```python
from build123d import *

# Parameters (mm, degrees)
SKETCH1_R           = 7.5
SKETCH1_R_2         = 4.1
BOSS_EXTRUDE1_DEPTH = 45
SKETCH2_R           = 6.75
SKETCH2_R_2         = 4.5
CUT_EXTRUDE2_DEPTH  = 0.75
CUT_EXTRUDE3_START  = -0.75
SKETCH3_R           = 7
SKETCH3_R_2         = 4.5
CUT_EXTRUDE3_DEPTH  = 0.75
SKETCH4_W           = 0.25
SKETCH4_H           = 1
SKETCH5_W           = 0.25
SKETCH5_H           = 1


with BuildPart() as part:
    # Sketch1 → Boss-Extrude1 (new body)
    with BuildSketch(Plane.XY):
        with Locations(Location((0, 0, 0), (0, 0, 180))):
            Circle(SKETCH1_R)
        with Locations(Location((0, 0, 0), (0, 0, 180))):
            Circle(SKETCH1_R_2, mode=Mode.SUBTRACT)
    extrude(amount=BOSS_EXTRUDE1_DEPTH)

    # Sketch2 → Cut-Extrude2 (cut)
    with BuildSketch(Plane.XY.offset(45)):
        Circle(SKETCH2_R)
        Circle(SKETCH2_R_2, mode=Mode.SUBTRACT)
    extrude(amount=-CUT_EXTRUDE2_DEPTH, mode=Mode.SUBTRACT)

    # Sketch3 → Cut-Extrude3 (cut)
    with BuildSketch(Plane(origin=(0, 0, 0), x_dir=(-1, 0, 0), z_dir=(0, 0, -1)).offset(CUT_EXTRUDE3_START)):
        Circle(SKETCH3_R)
        with Locations(Location((0, 0, 0), (0, 0, 180))):
            Circle(SKETCH3_R_2, mode=Mode.SUBTRACT)
    extrude(amount=CUT_EXTRUDE3_DEPTH, mode=Mode.SUBTRACT)

    # Sketch4 → Cut-Revolve1 (revolve, cut)
    with BuildSketch(Plane(origin=(0, 0, 0), x_dir=(1, 0, 0), z_dir=(0, 1, 0))):
        with Locations((-7.375, -39.5)):
            Rectangle(SKETCH4_W, SKETCH4_H)
    revolve(axis=Axis((0, 0, 45), (0, 0, -1)), mode=Mode.SUBTRACT)

    # Sketch5 → Cut-Revolve2 (revolve, cut)
    with BuildSketch(Plane(origin=(0, 0, 0), x_dir=(1, 0, 0), z_dir=(0, 1, 0))):
        with Locations((-7.375, -5.5)):
            Rectangle(SKETCH5_W, SKETCH5_H)
    revolve(axis=Axis((0, 0, 45), (0, 0, -1)), mode=Mode.SUBTRACT)


solid = part.part
```
CAD build for the part. Positions are in the model's coordinates, mm. A direction names the side the tool comes from. Give positions to 0.01 mm unless a question says otherwise; leave off trailing zeros. Loops run counter-clockwise (first coordinate to the right, second up) from the corner with the lowest first, then second, coordinate; pieces in that order, holes last. Notation, with made-up numbers: (-37.5, 78) -> (7.5, 78) arc R35 ccw to (7.5, 112) -> close; hole circle Ø6 at (43.5, 23). An arc over 180 degrees is marked (long way). Use a Markdown table: item, result.
1. Slice it at C-C (x = 6). List the corners of the cut face in (y, z), plus the area to 3 significant figures.
Check result:
| item | result |
|---|---|
| outline | (-4.5, 0) -> (-3.61, 0) -> (-3.61, 0.75) -> (3.61, 0.75) -> (3.61, 0) -> (4.5, 0) -> (4.5, 5) -> (4.07, 5) -> (4.07, 6) -> (4.5, 6) -> (4.5, 39) -> (4.07, 39) -> (4.07, 40) -> (4.5, 40) -> (4.5, 45) -> (3.09, 45) -> (3.09, 44.25) -> (-3.09, 44.25) -> (-3.09, 45) -> (-4.5, 45) -> (-4.5, 40) -> (-4.07, 40) -> (-4.07, 39) -> (-4.5, 39) -> (-4.5, 6) -> (-4.07, 6) -> (-4.07, 5) -> (-4.5, 5) -> close |
| area | 393 mm^2 |
2. Mould opens along Z. For faces 4 (the cylindrical face through (-4.032, -6.324, 2.465)), 5 (the flat face through (7, -1, 45)), 6 (the cylindrical face through (-3.35, -6.43, 5.49)) say: pulls with the +Z half, pulls with the -Z half, needs draft (parallel to the pull), parting line crosses it, or undercut.
Check result:
| item | result |
|---|---|
| face 4 | needs draft |
| face 5 | pulls with the +Z half |
| face 6 | undercut |
3. Slice it at A-A (z = 14). List the corners of the cut face in (x, y), plus the area to 3 significant figures.
Check result:
| item | result |
|---|---|
| outline | circle Ø15 at (0, 0); hole circle Ø8.2 at (0, 0) |
| area | 124 mm^2 |
4. Flat gauge pins, fed straight in: pin 1 (5 mm diameter, centred on y = -4.5, z = 33.5, fed in from -X); pin 2 (1 mm diameter, centred on x = 4.5, z = 24.5, fed in from +Y); pin 3 (3 mm diameter, centred on y = 3, z = 4.5, fed in from +X); pin 4 (1 mm diameter, centred on x = -2, y = 2, fed in from -Z). Where does each tip first touch, or does it go through?
Check result:
| item | result |
|---|---|
| pin 1 | stops at x = -7.23 |
| pin 2 | stops at y = 6.34 |
| pin 3 | stops at x = 7.35 |
| pin 4 | passes through |
5. Slice it at B-B (y = -5.75). List the corners of the cut face in (x, z), plus the area to 3 significant figures.
Check result:
| item | result |
|---|---|
| outline | (-4.82, 0) -> (-3.99, 0) -> (-3.99, 0.75) -> (3.99, 0.75) -> (3.99, 0) -> (4.82, 0) -> (4.82, 5) -> (4.42, 5) -> (4.42, 6) -> (4.82, 6) -> (4.82, 39) -> (4.42, 39) -> (4.42, 40) -> (4.82, 40) -> (4.82, 45) -> (3.54, 45) -> (3.54, 44.25) -> (-3.54, 44.25) -> (-3.54, 45) -> (-4.82, 45) -> (-4.82, 40) -> (-4.42, 40) -> (-4.42, 39) -> (-4.82, 39) -> (-4.82, 6) -> (-4.42, 6) -> (-4.42, 5) -> (-4.82, 5) -> close |
| area | 420 mm^2 |
6. Which spindle directions (+Z, -Z, +X, -X, +Y, -Y) get a long thin tool onto all of the face, cutting with end or side? Do faces 1 (the flat face through (4.4, 1.6, 44.25)), 2 (the flat face through (2, 7, 0)), 3 (the cylindrical face through (-6.466, -2.681, 0.38)). Say none if no direction does.
Check result:
| item | result |
|---|---|
| face 1 | +Z |
| face 2 | -Z, +X, -X, +Y, -Y |
| face 3 | -Z |
7. Wall check: L1, parallel to Y at x = 0, z = 0.25; L2, parallel to Y at x = 0, z = 44.6; L3, parallel to Y at x = 0, z = 30. Give the ranges that are in metal, low to high. Write a range as [from, to].
Check result:
| item | result |
|---|---|
| L1 | y = [-7.5, -7], [-4.5, -4.1], [4.1, 4.5], [7, 7.5] |
| L2 | y = [-7.5, -6.75], [-4.5, -4.1], [4.1, 4.5], [6.75, 7.5] |
| L3 | y = [-7.5, -4.1], [4.1, 7.5] |
